Verification items for the finished model (mm, model axes). A direction names the side the tool comes from. Coordinates: 2 decimals unless noted, no trailing zeros. Order: outer loops, then holes, each group sorted by start corner. A loop starts at its lowest first (then second) coordinate and runs counter-clockwise, first axis right, second up. Notation, with made-up numbers: (-33.5, 18.5) - (-4.5, 18.5) arc R6 cw to (-4.5, 25.5) - close; hole circle Ø2 at (11.5, 7). An arc over 180 degrees is marked (long way). Answer as CSV lines item,"result". Start each with the question number.
1. Section check B-B (y = 13). Record the cut outline in (x, z).
2. Material ranges on L1, parallel to Y at x = 9, z = 8; L2, parallel to X at y = 26.5, z = 17.5; L3, parallel to Y at x = 27, z = 8, recorded low to high. Write a range as [from, to].
3. Section check D-D (y = -3.5). Record the cut outline in (x, z).
4. Set-up check for faces 1 (the flat face through (0, -61, 9)), 2 (the flat face through (0, 1, 20)): record each of +Z, -Z, +X, -X, +Y, -Y from which the full face is reachable in a straight line by a thin tool's end or side.
5. Go/stop test with a flat-tipped pin: pin 1 (5 mm diameter, centred on x = -23, y = -10.5, fed in from -Z). Record where the tip stops, or that it passes through.
6. Section check A-A (z = 2). Record the cut outline in (x, y).
7. Section check C-C (x = -10.5). Record the cut outline in (y, z), and give its area (3 significant figures).
8. Mould release check, pull along X, two halves, no side actions. Record for faces 3 (the flat face through (0, -62.5, 10)), 4 (the flat face through (-30, -1, 10)), 5 (the cylindrical face through (-27.297, -59.859, 9.38)): pulls with the +X half, pulls with the -X half, needs draft (parallel to the pull), parting line crosses it, or undercut.
from build123d import *

# Parameters (mm, degrees)
F0_W     = 60
F0_H     = 125
F1_DEPTH = 20
F2_W     = 57
F2_H     = 60.25
F3_DEPTH = 18.5
F4_R     = 4


with BuildPart() as f1:
    # F0 (on Top) → F1 (new body)
    with BuildSketch(Plane.XY):
        Rectangle(F0_W, F0_H)
    extrude(amount=F1_DEPTH)

    # F2 (on Top) → F3 (cut)
    with BuildSketch(Plane.XY):
        with Locations((0, 30.875)):
            Rectangle(F2_W, F2_H)
        with Locations((0, -30.875)):
            Rectangle(F2_W, F2_H)
    extrude(amount=F3_DEPTH, mode=Mode.SUBTRACT)

    # F4
    f4_edges = [f1.edges().sort_by_distance(p)[0] for p in [
        (28.5, -61, 9.25),
        (28.5, 0.75, 9.25),
        (-28.5, -61, 9.25),
        (-28.5, 0.75, 9.25),
        (-28.5, -0.75, 9.25),
        (-28.5, 61, 9.25),
        (28.5, 61, 9.25),
        (28.5, -0.75, 9.25),
    ]]
    fillet(f4_edges, radius=F4_R)


solid = f1.part
Evaluation:
1,outline,"(-30, 0) - (-28.5, 0) - (-28.5, 18.5) - (28.5, 18.5) - (28.5, 0) - (30, 0) - (30, 20) - (-30, 20) - close"
2,L1,"y = [-62.5, -61], [-0.75, 0.75], [61, 62.5]"
2,L2,"x = [-30, -28.5], [28.5, 30]"
2,L3,"y = [-62.5, -60.12], [-1.63, 1.63], [60.12, 62.5]"
3,outline,"(-30, 0) - (-28.3, 0) - (-28.3, 18.5) - (28.3, 18.5) - (28.3, 0) - (30, 0) - (30, 20) - (-30, 20) - close"
4,face 1,"-Z"
4,face 2,"+Z, +X, -X, +Y, -Y"
5,pin 1,"stops at z = 18.5"
6,outline,"(-30, -62.5) - (30, -62.5) - (30, 62.5) - (-30, 62.5) - close; hole (-28.5, -57) arc R4 ccw to (-24.5, -61) - (24.5, -61) arc R4 ccw to (28.5, -57) - (28.5, -4.75) arc R4 ccw to (24.5, -0.75) - (-24.5, -0.75) arc R4 ccw to (-28.5, -4.75) - close; hole (-28.5, 4.75) arc R4 ccw to (-24.5, 0.75) - (24.5, 0.75) arc R4 ccw to (28.5, 4.75) - (28.5, 57) arc R4 ccw to (24.5, 61) - (-24.5, 61) arc R4 ccw to (-28.5, 57) - close"
7,outline,"(-62.5, 0) - (-61, 0) - (-61, 18.5) - (-0.75, 18.5) - (-0.75, 0) - (0.75, 0) - (0.75, 18.5) - (61, 18.5) - (61, 0) - (62.5, 0) - (62.5, 20) - (-62.5, 20) - close"
7,area,"271 mm²"
8,face 3,"needs draft"
8,face 4,"pulls with the -X half"
8,face 5,"undercut"
